Design review of the part built by this model. Coordinates are the model's own, in mm. A direction names the side the tool comes from. Round coordinates to 2 decimals unless told otherwise and drop trailing zeros. Order: outer loops, then holes, each group sorted by start corner. A loop starts at its lowest first (then second) coordinate and runs counter-clockwise, first axis right, second up.
from build123d import *

# Parameters (mm, degrees)
EXTRUDE_1_DEPTH = 8
EXTRUDE_2_DEPTH = 10


with BuildPart() as part:
    # 草图1 → 凸台-拉伸1 (new body)
    with BuildSketch(Plane.XY):
        with BuildLine():
            Line((0, 15.5), (0, -15.5))
            ThreePointArc((0, -15.5), (-3.872839431, -15.008368157), (-7.5, -13.564659966))
            Line((-7.5, -13.564659966), (-7.5, 13.564659966))
            ThreePointArc((-7.5, 13.564659966), (-3.872839431, 15.008368157), (0, 15.5))
        make_face()
    extrude(amount=EXTRUDE_1_DEPTH)

    # 草图2 → 凸台-拉伸2 (add)
    with BuildSketch(Plane.XY.offset(8)):
        with BuildLine():
            Line((7.5, 5), (9.5, 5))
            Line((9.5, 5), (9.5, 15))
            Line((9.5, 15), (-9.5, 15))
            Line((-9.5, 15), (-9.5, 5))
            Line((-9.5, 5), (-7.5, 5))
            ThreePointArc((-7.5, 5), (0, 12.5), (7.5, 5))
        make_face()
    extrude(amount=EXTRUDE_2_DEPTH)


solid = part.part
1) For faces 4 (the face through (-0.16, 12.5, 12.93)), 5 (the face through (-9, 11, 8)), 6 (the face through (-7.5, 0, 4)), list the 3-axis set-ups (+Z, -Z, +X, -X, +Y, -Y) from which the entire face can be reached by the end or side of a thin tool; tool diameter is ignored.
Results:
face 4: +Z, -Y
face 5: -Z, -X, +Y
face 6: -Z, -X, +Y, -Y
2) Clearance check with flat-ended pins moving along their axes: P1, Ø8, axis at y = -8, z = 13, coming from the -X side; P2, Ø4, axis at x = -2, y = -0.5, coming from the +Z side; P3, Ø3, axis at x = -5, z = 9, coming from the -Y side; P4, Ø0.6, axis at x = -8.5, z = 12, coming from the -Y side. State where each tip first meets the part, or that it passes through.
Results:
P1: passes through
P2: stops at z = 8
P3: stops at y = -15.01
P4: stops at y = 5
3) Take a section at A-A on y = 11. Give the boundary of the cut face in (x, z), plus the area to 3 significant figures.
Results:
outline: (-9.5, 8) - (-7.5, 8) - (-7.5, 0) - (0, 0) - (0, 8) - (-4.5, 8) - (-4.5, 18) - (-9.5, 18) - close; (4.5, 8) - (9.5, 8) - (9.5, 18) - (4.5, 18) - close
area: 160 mm2
4) Take a section at B-B on z = 8.5. Give the boundary of the cut face in (x, y).
Results:
outline: (-9.5, 5) - (-7.5, 5) arc R7.5 cw to (7.5, 5) - (9.5, 5) - (9.5, 15) - (-9.5, 15) - close
5) To check wall thickness, follow line 1 along X through (y, z) = (-2.5, 7.25); line 2 along Z through (x, y) = (-5, 4); line 3 along Z through (x, y) = (6, 10). State the ranges of each line that lie inside material, in increasing order.
Results:
line 1: x = -7.5 to 0
line 2: z = 0 to 8
line 3: z = 8 to 18
6) Take a section at C-C on x = -3.5. Give the boundary of the cut face in (y, z), plus the area to 3 significant figures.
Results:
outline: (-15.1, 0) - (15.1, 0) - (15.1, 8) - (15, 8) - (15, 18) - (11.63, 18) - (11.63, 8) - (-15.1, 8) - close
area: 275 mm2
7) Take a section at D-D on y = -1.5. Give the boundary of the cut face in (x, z).
Results:
outline: (-7.5, 0) - (0, 0) - (0, 8) - (-7.5, 8) - close
8) The part is to be moulded in two halves that separate along X. For faces 1 (the face through (6, 11, 8)), 2 (the face through (-4, -1, 8)), 3 (the face through (-3.82, -15.02, 3.94)), say which applies: released by +X, released by -X, zero draft, split by the parting line, or undercut.
Results:
face 1: zero draft
face 2: undercut
face 3: released by -X
